Geometry check sheet. Reference: the model listing, model coordinates, mm. A direction names the side the tool comes from. Round coordinates to 2 decimals unless told otherwise and drop trailing zeros. Order: outer loops, then holes, each group sorted by start corner. A loop starts at its lowest first (then second) coordinate and runs counter-clockwise, first axis right, second up. Notation, with made-up numbers: (-27, 41.25) -> (27, 41.25) arc R18 ccw to (27, 72.25) -> close; hole circle Ø9 at (65, -16.75). An arc over 180 degrees is marked (long way). Use a Markdown table: item, result. Add a question column.
Item 1: Material ranges on probe 1 along Y at (x, z) = (-0.5, 19.5); probe 2 along Z at (x, y) = (0, -4.55), recorded low to high. Write a range as [from, to].
Item 2: Sectioned sample at A-A, the plane x = 3. Record the cut outline in (y, z).
Item 3: Set-up check for faces 4 (the flat face through (5, 0, 20)), 5 (the flat face through (0, -3.5, 20)): record each of +Z, -Z, +X, -X, +Y, -Y from which the full face is reachable in a straight line by a thin tool's end or side.
Item 4: Sectioned sample at D-D, the plane z = 35. Record the cut outline in (x, y).
Item 5: Mould release check, pull along Z, two halves, no side actions. Record for faces 1 (the cylindrical face through (0.46, -4.26, 37.05)), 2 (the flat face through (-4.5, 0.1, 0)), 3 (the flat face through (3.5, 0, 20)): pulls with the +Z half, pulls with the -Z half, needs draft (parallel to the pull), parting line crosses it, or undercut.
Item 6: Sectioned sample at C-C, the plane x = 0. Record the cut outline in (y, z), and give its area (3 significant figures).
from build123d import *

# Parameters (mm, degrees)
SKETCH_1_W         = 10
SKETCH_1_H         = 10
SKETCH_1_W_2       = 7
SKETCH_1_H_2       = 7
EXTRUDE_1_DEPTH    = 40
HOLE_WIZARD_M5_1_D = 4.2


with BuildPart() as part:
    # 草圖1 → 伸長-薄件1 (new body)
    with BuildSketch(Plane.XY):
        Rectangle(SKETCH_1_W, SKETCH_1_H)
        Rectangle(SKETCH_1_W_2, SKETCH_1_H_2, mode=Mode.SUBTRACT)
    extrude(amount=EXTRUDE_1_DEPTH)

    # M5 螺紋孔1 (through all)
    with Locations(Plane(origin=(0, 5, 0), x_dir=(1, 0, 0), z_dir=(0, 1, 0))):
        with Locations((0, -35)):
            Hole(HOLE_WIZARD_M5_1_D / 2)


solid = part.part
Found:
| question | item | result |
|---|---|---|
| 1 | probe 1 | y = [-5, -3.5], [3.5, 5] |
| 1 | probe 2 | z = [0, 32.9], [37.1, 40] |
| 2 | outline | (-5, 0) -> (-3.5, 0) -> (-3.5, 40) -> (-5, 40) -> close; (3.5, 0) -> (5, 0) -> (5, 40) -> (3.5, 40) -> close |
| 3 | face 4 | +Z, -Z, +X, +Y, -Y |
| 3 | face 5 | +Z, -Z |
| 4 | outline | (-5, -5) -> (-2.1, -5) -> (-2.1, -3.5) -> (-3.5, -3.5) -> (-3.5, 3.5) -> (-2.1, 3.5) -> (-2.1, 5) -> (-5, 5) -> close; (2.1, -5) -> (5, -5) -> (5, 5) -> (2.1, 5) -> (2.1, 3.5) -> (3.5, 3.5) -> (3.5, -3.5) -> (2.1, -3.5) -> close |
| 5 | face 1 | undercut |
| 5 | face 2 | pulls with the -Z half |
| 5 | face 3 | needs draft |
| 6 | outline | (-5, 0) -> (-3.5, 0) -> (-3.5, 32.9) -> (-5, 32.9) -> close; (-5, 37.1) -> (-3.5, 37.1) -> (-3.5, 40) -> (-5, 40) -> close; (3.5, 0) -> (5, 0) -> (5, 32.9) -> (3.5, 32.9) -> close; (3.5, 37.1) -> (5, 37.1) -> (5, 40) -> (3.5, 40) -> close |
| 6 | area | 107 mm2 |
